Source: CAD feature listing. Evaluate the final solid. Frame: model axes, mm. Face numbers are marked on the shaded views. A direction names the side the tool comes from. Round coordinates to 2 decimals unless told otherwise and drop trailing zeros. Write each loop counter-clockwise with the first axis right and the second up, starting at its lowest first coordinate (ties: lowest second). Pieces come first, ordered by that corner, then holes. Notation, with made-up numbers: M 6.25,3 L 18.25,3 A21 ccw 18.25,33 Z; hole C -16.75,70 d2. An arc over 180 degrees is marked long. Answer in a Markdown table with one row per item.
from build123d import *

# Parameters (mm, degrees)
SKETCH_2_W          = 1
SKETCH_2_H          = 1
CUT_EXTRUDE_1_DEPTH = 5


with BuildPart() as part:
    # Эскиз1 → Повернуть1 (revolve)
    with BuildSketch(Plane.XY, mode=Mode.PRIVATE) as revolve_1_sk:
        with BuildLine():
            Line((0, 0), (0, 8.12))
            Line((0, 8.12), (1.25, 8.12))
            ThreePointArc((1.25, 8.12), (2.310660172, 7.680660172), (2.75, 6.62))
            Line((2.75, 6.62), (2.75, 6))
            Line((2.75, 6), (1.5, 6))
            Line((1.5, 6), (1.5, 2.9))
            Line((1.5, 2.9), (1.367139057, 1))
            Line((1.367139057, 1), (1.172758748, 0))
            Line((1.172758748, 0), (0, 0))
        make_face()
    revolve(revolve_1_sk.sketch.rotate(Axis((0, 0, 0), (0, 1, 0)), 90), axis=Axis((0, 0, 0), (0, 1, 0)))

    # Эскиз2 → Вырез-Вытянуть1 (cut, symmetric)
    with BuildSketch(Plane(origin=(0, 0, 0), x_dir=(0, 0, -1), z_dir=(1, 0, 0))):
        with Locations((0, 7.62)):
            Rectangle(SKETCH_2_W, SKETCH_2_H)
    extrude(amount=CUT_EXTRUDE_1_DEPTH, both=True, mode=Mode.SUBTRACT)


solid = part.part
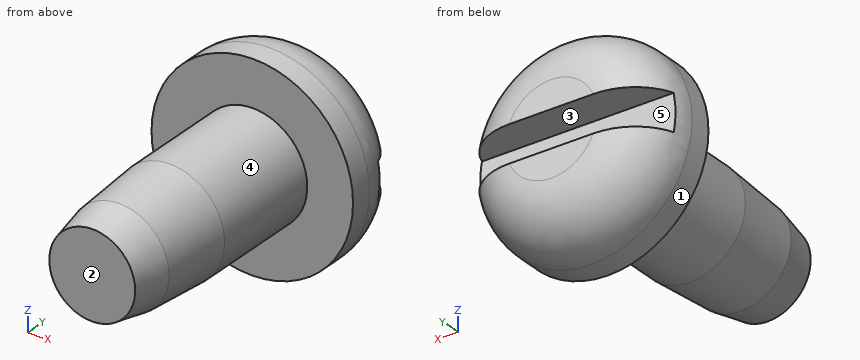
Q1. Section B-B (y = 2). Return loops of the section in (x, z).
Solutions:
| item | result |
|---|---|
| outline | C 0,0 d2.87 |
Q2. Section A-A (y = 5). Return loops of the section in (x, z).
Solutions:
| item | result |
|---|---|
| outline | C 0,0 d3 |
Q3. Contact query for flat-ended pins moving along their axis: pin 1 Ø2 at (x, y) = (0, 4) entering from +Z; pin 2 Ø1 at (x, z) = (1.5, 1.5) entering from -Y; pin 3 Ø1.1 at (x, y) = (-0.5, 7.5) entering from -Z. Output: stop coordinate, or through.
Solutions:
| item | result |
|---|---|
| pin 1 | stops at z = 1.5 |
| pin 2 | stops at y = 6 |
| pin 3 | stops at z = -2.69 |
Q4. Pull-direction query (Z, two-part tool) for the marked faces 1, 2 and 3; classes: pulls with the +Z half, pulls with the -Z half, needs draft (parallel to the pull), parting line crosses it, or undercut.
Solutions:
| item | result |
|---|---|
| face 1 | parting line crosses it |
| face 2 | needs draft |
| face 3 | undercut |
Q5. Access query for the marked faces 4 and 5. Directions: +Z, -Z, +X, -X, +Y, -Y. A direction counts if a zero-diameter tool reaches every point of the face in a straight line with its end or side. Return the directions, or none.
Solutions:
| item | result |
|---|---|
| face 4 | -Y |
| face 5 | +X, -X, +Y |
Q6. Material intervals for probe 1 along Y at (x, z) = (0.1, -0.2); probe 2 along Z at (x, y) = (-0.4, 7.5); probe 3 along Y at (x, z) = (-1.9, -0.45), sorted ascending.
Solutions:
| item | result |
|---|---|
| probe 1 | y = 0 to 7.12 |
| probe 2 | z = -2.43 to -0.5, 0.5 to 2.43 |
| probe 3 | y = 6 to 7.12 |
